Here's how the part is built. I have some questions about the finished solid (model axes, mm). Coordinates: 2 decimals unless noted, no trailing zeros. Loops run counter-clockwise (first coordinate to the right, second up) from the corner with the lowest first, then second, coordinate; pieces in that order, holes last. Notation, with made-up numbers: M 52,25 L 100,25 A14 ccw 100,31 Z; hole C -19.5,44.25 d2. An arc over 180 degrees is marked long. Use one line per item in the form item = value. Start each with the question number.
(1) Please list where these lines run through material, in increasing order: L1, parallel to Z at x = -57, y = 30; L2, parallel to Z at x = -6, y = 10.5; L3, parallel to X at y = -1, z = 56.
(2) Imagine slicing it at C-C, the plane x = -38.1. Please give me the cut outline in (y, z), and give its area (3 significant figures).
(3) Will these pins go through, and if not, where does the flat tip stop? P1, Ø4, axis at y = 7.5, z = 15.5, coming from the -X side; P2, Ø2, axis at x = -46, y = 20.5, coming from the -Z side; P3, Ø10, axis at y = -6, z = 78.5, coming from the -X side; P4, Ø6, axis at x = -66, y = -24.5, coming from the -Z side.
(4) Imagine slicing it at D-D, the plane z = 17. Please give me the cut outline in (x, y).
(5) Imagine slicing it at A-A, the plane y = 0. Please give me the cut outline in (x, z), and give its area (3 significant figures).
(6) Imagine slicing it at B-B, the plane z = 71. Please give me the cut outline in (x, y), and give its area (3 significant figures).
```python
from build123d import *


# Not quite as in the source:
# - a fillet or chamfer that OpenCascade refuses, or shapes differently, is made with other operations: its cross-section is extruded or revolved along the edge and cut away or added


with BuildPart() as f1:
    # F0 (on Front) → F1 (revolve)
    with BuildSketch(Plane.XZ):
        with BuildLine():
            Line((-38.1, 0), (0, 0))
            Line((0, 0), (0, 19.05))
            ThreePointArc((0, 19.05), (-6.35, 25.4), (0, 31.75))
            Line((0, 31.75), (0, 95.25))
            ThreePointArc((0, 95.25), (-6.35, 101.6), (0, 107.95))
            Line((0, 107.95), (0, 127))
            Line((0, 127), (-38.1, 127))
            Line((-38.1, 127), (-38.1, 0))
        make_face()
    revolve(axis=Axis((-38.1, 0, 63.5), (0, 0, 1)))

    # F2: chamfer of 5.08 on 4 edges, made by hand

    # F2_s1 → F2_t2 (revolve, cut)
    with BuildSketch(Plane.XZ):
        Polygon((0, 121.92), (-5.08, 127), (0, 127), align=None)
    revolve(axis=Axis((-38.1, 0, 127), (0, 0, 1)), mode=Mode.SUBTRACT)

    # F2_s3 → F2_t4 (revolve, cut)
    with BuildSketch(Plane.XZ):
        Polygon((-5.08, 0), (0, 5.08), (0, 0), align=None)
    revolve(axis=Axis((-38.1, 0, 0), (0, 0, 1)), mode=Mode.SUBTRACT)

    # F2_s5 → F2_t6 (revolve, cut)
    with BuildSketch(Plane.XZ):
        with BuildLine():
            Line((0, 15.1609326597), (-2.8222222222, 19.7116292554))
            ThreePointArc((-2.8222222222, 19.7116292554), (-1.5219513398, 19.2350860412), (0, 19.05))
            Line((0, 19.05), (0, 15.1609326597))
        make_face()
    revolve(axis=Axis((-38.1, 0, 19.05), (0, 0, 1)), mode=Mode.SUBTRACT)


solid = f1.part
```
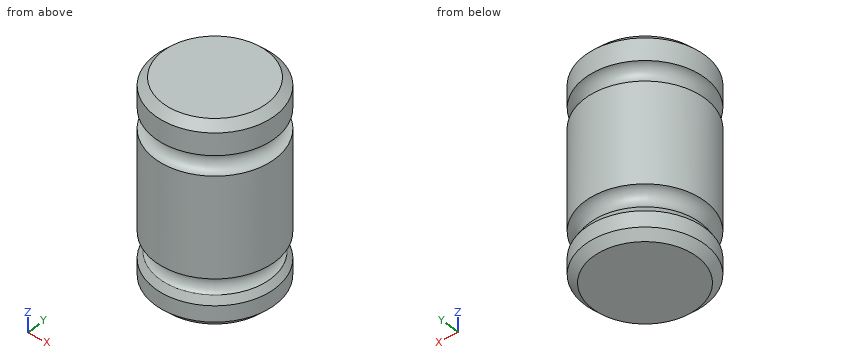
Answer:
q1.L1 = 2.44 to 19.42, 31.17 to 95.83, 107.37 to 124.56
q1.L2 = 0.75 to 20.75, 30.05 to 96.95, 106.25 to 126.25
q1.L3 = -76.19 to -0.01
q2.outline = M -38.1,5.08 L -33.02,0 L 33.02,0 L 38.1,5.08 L 38.1,15.16 L 35.28,19.71 A6.35 cw 38.1,31.75 L 38.1,95.25 A6.35 cw 38.1,107.95 L 38.1,121.92 L 33.02,127 L -33.02,127 L -38.1,121.92 L -38.1,107.95 A6.35 cw -38.1,95.25 L -38.1,31.75 A6.35 cw -35.28,19.71 L -38.1,15.16 Z
q2.area = 9,360 mm²
q3.P1 = -75.8
q3.P2 = 0
q3.P3 = -76.19
q3.P4 = 1.11
q4.outline = C -38.1,0 d73.92
q5.outline = M -76.2,5.08 L -71.12,0 L -5.08,0 L 0,5.08 L 0,15.16 L -2.82,19.71 A6.35 cw 0,31.75 L 0,95.25 A6.35 cw 0,107.95 L 0,121.92 L -5.08,127 L -71.12,127 L -76.2,121.92 L -76.2,107.95 A6.35 cw -76.2,95.25 L -76.2,31.75 A6.35 cw -73.38,19.71 L -76.2,15.16 Z
q5.area = 9,360 mm²
q6.outline = C -38.1,0 d76.2
q6.area = 4,560 mm²
